Check sheet for the drawn part. Datum: minimum x, y, z corner. Units: mm. A direction names the side the tool comes from. Give positions to 0.01 mm unless a question says otherwise; leave off trailing zeros. Write each loop counter-clockwise with the first axis right and the second up, starting at its lowest first coordinate (ties: lowest second). Pieces come first, ordered by that corner, then holes.
(1) Cross-section at A-A (x = 36). Record the boundary of the cut face in (y, z).
(2) Cross-section at B-B (y = 16). Record the boundary of the cut face in (x, z).
(3) Cross-section at D-D (y = 53). Record the boundary of the cut face in (x, z), and give its area (3 significant figures).
(4) Tool access check on the marked faces 1 and 2. Record the directions out of +Z, -Z, +X, -X, +Y, -Y that give a thin tool (end or side, any length) a straight path to the whole face; none if there is none.
(5) Thickness scan on line 1 along Y through (x, z) = (36, 2.15); line 2 along Z through (x, y) = (21.5, 14); line 3 along X through (y, z) = (84.5, 42). Record the ranges inside material, lowest first.
(6) Cross-section at C-C (z = 9.5). Record the boundary of the cut face in (x, y) (1 decimal), and give its area (3 significant figures).
(7) Depth check by flat-ended pin: P1, Ø5, axis at y = 37, z = 13, coming from the -X side; P2, Ø6, axis at y = 64.5, z = 38, coming from the -X side; P3, Ø2, axis at y = 23, z = 13, coming from the +X side. Enter the tip coordinate at first touch or a pass-through.
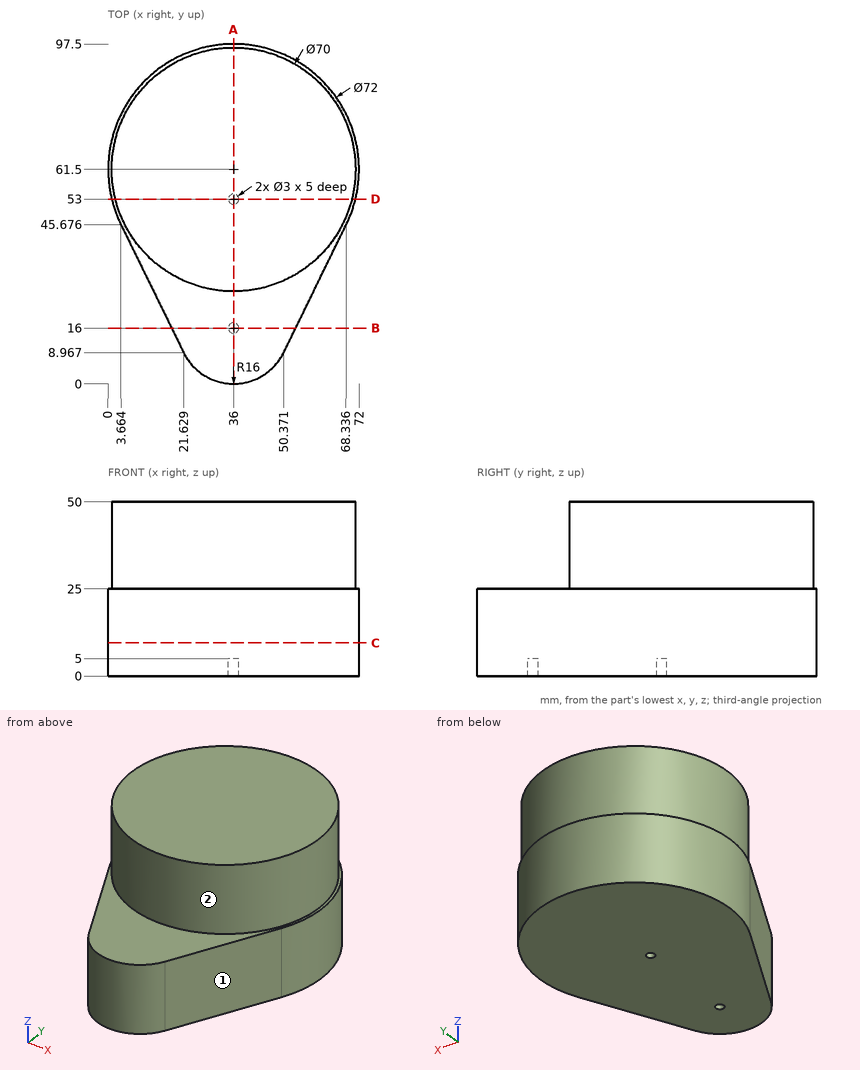
Reply:
1. outline: (0, 0) - (14.5, 0) - (14.5, 5) - (17.5, 5) - (17.5, 0) - (51.5, 0) - (51.5, 5) - (54.5, 5) - (54.5, 0) - (97.5, 0) - (97.5, 25) - (96.5, 25) - (96.5, 50) - (26.5, 50) - (26.5, 25) - (0, 25) - close
2. outline: (18.19, 0) - (34.5, 0) - (34.5, 5) - (37.5, 5) - (37.5, 0) - (53.81, 0) - (53.81, 25) - (18.19, 25) - close
3. outline: (1.02, 0) - (34.5, 0) - (34.5, 5) - (37.5, 5) - (37.5, 0) - (70.98, 0) - (70.98, 25) - (69.95, 25) - (69.95, 50) - (2.05, 50) - (2.05, 25) - (1.02, 25) - close
3. area: 3,430 mm2
4. face 1: +Z, -Z, +X, -Y
4. face 2: +Z
5. line 1: y = 0 to 14.5, 17.5 to 51.5, 54.5 to 97.5
5. line 2: z = 0 to 25
5. line 3: x = 9.62 to 62.38
6. outline: (3.7, 45.7) - (21.6, 9) arc R16 ccw to (50.4, 9) - (68.3, 45.7) arc R36 ccw (long way) to start
6. area: 5,040 mm2
7. P1: stops at x = 6.69
7. P2: stops at x = 1
7. P3: stops at x = 57.73
